Study the drawing (mm; zero at the part's minimum x, y, z) and answer. Give positions to 0.01 mm unless a question says otherwise; leave off trailing zeros. Order: outer loops, then holes, each group sorted by start corner. A loop starts at its lowest first (then second) coordinate and runs counter-clockwise, first axis right, second up. Notation, with made-up numbers: (-8, 58) - (50, 58) arc R25 cw to (50, 91) - close; hole circle Ø3 at (-26, -27.75). An arc over 180 degrees is marked (long way). Write each question's results on one line, items separated by ' | '. Start each with the question number.
Q1. Find section B-B on y = 75. Give the vertices of the cut face in (x, z).
Q2. Find the intervals of material crossed by line 1 along Y through (x, z) = (7, 75); line 2 along Z through (x, y) = (8, 94.5); line 3 along Y through (x, z) = (5.5, 116), in increasing order. Write a range as from..to.
Q3. Find section C-C on z = 42.5. Give the vertices of the cut face in (x, y), and give its area (3 significant figures).
Q4. A flat-ended cylindrical pin translates along its axis: P1, Ø19, axis at y = 113.73, z = 75, coming from the +X side (3 decimals). Find the tip coordinate at first contact, or state that the pin passes through.
Q5. Find section D-D on x = 8. Give the vertices of the cut face in (y, z).
Q6. Find section A-A on z = 75. Give the vertices of the cut face in (x, y).
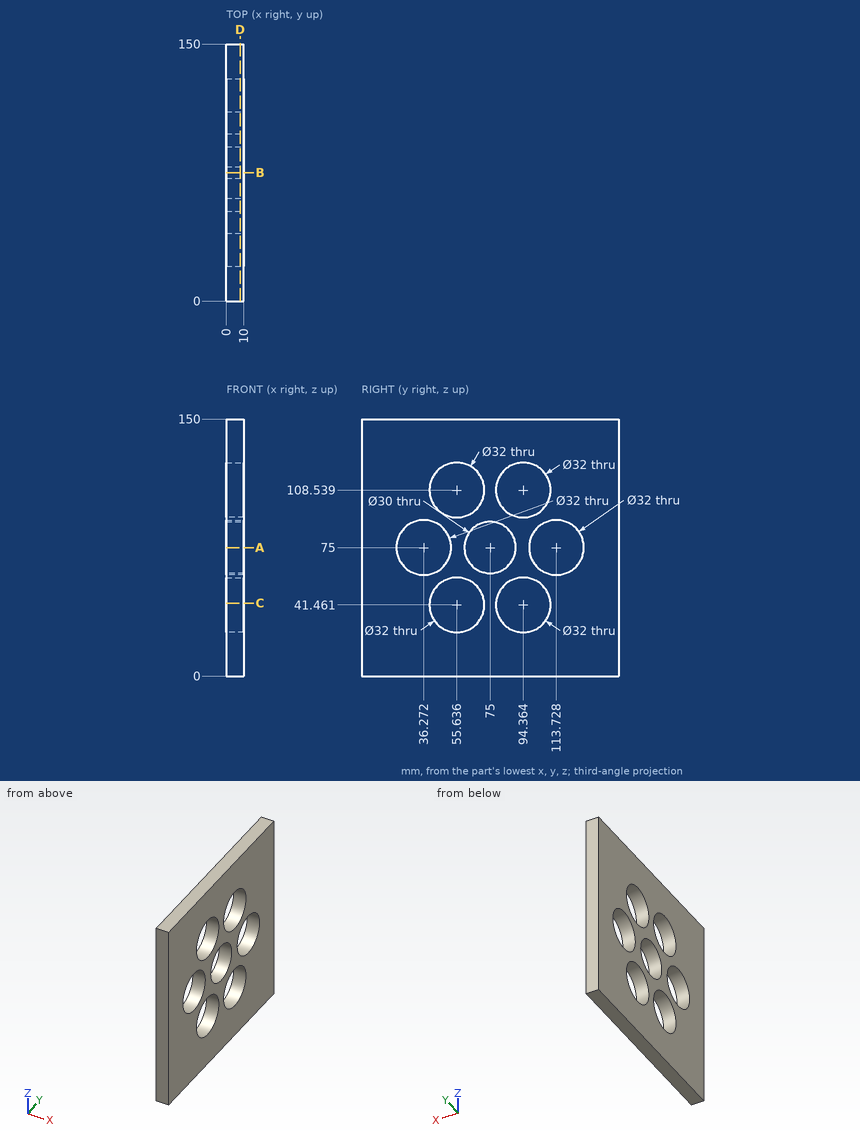
Working result:
1) outline: (0, 0) - (10, 0) - (10, 60) - (0, 60) - close; (0, 90) - (10, 90) - (10, 150) - (0, 150) - close
2) line 1: 0..20.27, 52.27..60, 90..97.73, 129.73..150 | line 2: 0..25.46, 57.46..92.54, 124.54..150 | line 3: 0..41.48, 69.79..80.21, 108.52..150
3) outline: (0, 0) - (10, 0) - (10, 39.67) - (0, 39.67) - close; (0, 71.6) - (10, 71.6) - (10, 78.4) - (0, 78.4) - close; (0, 110.33) - (10, 110.33) - (10, 150) - (0, 150) - close | area: 861 mm²
4) P1: through
5) outline: (0, 0) - (150, 0) - (150, 150) - (0, 150) - close; hole circle Ø32 at (36.27, 75); hole circle Ø32 at (55.64, 41.46); hole circle Ø32 at (55.64, 108.54); hole circle Ø30 at (75, 75); hole circle Ø32 at (94.36, 41.46); hole circle Ø32 at (94.36, 108.54); hole circle Ø32 at (113.73, 75)
6) outline: (0, 0) - (10, 0) - (10, 20.27) - (0, 20.27) - close; (0, 52.27) - (10, 52.27) - (10, 60) - (0, 60) - close; (0, 90) - (10, 90) - (10, 97.73) - (0, 97.73) - close; (0, 129.73) - (10, 129.73) - (10, 150) - (0, 150) - close
